Work out the finished part from the listing and answer in its coordinate system (mm). A direction names the side the tool comes from. Round coordinates to 2 decimals unless told otherwise and drop trailing zeros. Order: outer loops, then holes, each group sorted by start corner. A loop starts at its lowest first (then second) coordinate and runs counter-clockwise, first axis right, second up. Notation, with made-up numbers: (36, -21.75) -> (54, -21.75) arc R10 cw to (54, -2.75) -> close; hole circle Ø4 at (0.25, -31.75). An arc over 180 degrees is marked (long way). Use a Markdown table: item, result. Add a question column.
Item 1: Find the intervals of material crossed by L1, parallel to Z at x = 215, y = 18, in increasing order. Write a range as [from, to].
Item 2: A tool of negligible diameter and unlimited length cuts with its end or side. For faces 4 (the flat face through (216, 0, 17)), 5 (the flat face through (215, 15, -2)), 6 (the flat face through (215, -17, 35)), 7 (the flat face through (215, -15, -2)), 8 (the flat face through (215, 17, 35)), from which of +Z, -Z, +X, -X, +Y, -Y can it reach the whole face along a straight path? Write none if from no direction.
Item 3: Flat-ended cylindrical pins translate along their axes: P1, Ø1, axis at x = 215, y = -18.5, coming from the -Z side; P2, Ø1, axis at x = 215.5, z = -1, coming from the -Y side; P3, Ø0.6, axis at x = 215.5, y = -17.5, coming from the +Z side. Find the tip coordinate at first contact, or state that the pin passes through.
Item 4: For a pull along Y with two mould halves and no side action, classify faces 1 (the flat face through (215, 20, 18)), 2 (the flat face through (214, 0, 17)), 3 (the flat face through (215, -15, 36)) as +Y half, -Y half, draft (parallel to the pull), parting line (faces both ways), or undercut.
Item 5: A cutting plane is placed at A-A, the plane x = 214.45. Determine the outline of the cut face in (y, z).
from build123d import *

# Parameters (mm, degrees)
ESTRUSIONE_ESTRUSIONE1_DEPTH      = 37
ESTRUSIONE_ESTRUSIONE1_DEPTH_BACK = 3
SCHIZZO1_W                        = 2
SCHIZZO1_H                        = 30
SCHIZZO2_W                        = 2
SCHIZZO2_H                        = 35
ESTRUSIONE_ESTRUSIONE2_DEPTH      = 5


with BuildPart() as part:
    # Schizzo1 → Estrusione-Estrusione1 (new, two sides: drawn at the far end of the back side and taken through both)
    with BuildSketch(Plane.XY.offset(-ESTRUSIONE_ESTRUSIONE1_DEPTH_BACK)):
        with Locations((215, 0)):
            Rectangle(SCHIZZO1_W, SCHIZZO1_H)
    extrude(amount=ESTRUSIONE_ESTRUSIONE1_DEPTH + ESTRUSIONE_ESTRUSIONE1_DEPTH_BACK)

    # Schizzo2 → Estrusione-Estrusione2 (add)
    with BuildSketch(Plane.XZ.offset(15)):
        with Locations((215, 17.5)):
            Rectangle(SCHIZZO2_W, SCHIZZO2_H)
    estrusione_estrusione2 = extrude(amount=ESTRUSIONE_ESTRUSIONE2_DEPTH)

    # Specchia1: Estrusione-Estrusione2 across plane
    add(estrusione_estrusione2.mirror(Plane.ZX))


solid = part.part
Reported:
| question | item | result |
|---|---|---|
| 1 | L1 | [0, 35] |
| 2 | face 4 | +Z, -Z, +X, +Y, -Y |
| 2 | face 5 | -Z, +X, -X, +Y |
| 2 | face 6 | +Z, +X, -X, -Y |
| 2 | face 7 | -Z, +X, -X, -Y |
| 2 | face 8 | +Z, +X, -X, +Y |
| 3 | P1 | z = 0 |
| 3 | P2 | y = -15 |
| 3 | P3 | z = 35 |
| 4 | face 1 | +Y half |
| 4 | face 2 | draft |
| 4 | face 3 | -Y half |
| 5 | outline | (-20, 0) -> (-15, 0) -> (-15, -3) -> (15, -3) -> (15, 0) -> (20, 0) -> (20, 35) -> (15, 35) -> (15, 37) -> (-15, 37) -> (-15, 35) -> (-20, 35) -> close |
